from build123d import *

# Parameters (mm, degrees)
F0_W     = 60.3929003701
F0_H     = 33.9642912149
F1_DEPTH = 35.814
F2_T     = 2.54


with BuildPart() as f1:
    # F0 (on Front) → F1 (new body)
    with BuildSketch(Plane.XZ):
        with Locations((-40.0745426305, 29.1485004127)):
            Rectangle(F0_W, F0_H)
    extrude(amount=F1_DEPTH)

    # F2 (hollow, outwards: the wall grows on the outside; the body as it was is the cavity)
    f2_inside = f1.part
    offset(amount=F2_T, kind=Kind.INTERSECTION)
    add(f2_inside, mode=Mode.SUBTRACT)


solid = f1.part
Verification items for the finished model (mm, model axes). A direction names the side the tool comes from. Coordinates: 2 decimals unless noted, no trailing zeros. Order: outer loops, then holes, each group sorted by start corner. A loop starts at its lowest first (then second) coordinate and runs counter-clockwise, first axis right, second up.
Item 1: Section check B-B, the plane y = -7.5. Enter the section's corners in (x, z).
Filled in:
outline: (-72.81, 9.63) - (-7.34, 9.63) - (-7.34, 48.67) - (-72.81, 48.67) - close; hole (-70.27, 12.17) - (-9.88, 12.17) - (-9.88, 46.13) - (-70.27, 46.13) - close
Item 2: Section check A-A, the plane x = -26.5. Enter the section's corners in (y, z), then the cut area to 3 significant figures.
Filled in:
outline: (-38.35, 9.63) - (2.54, 9.63) - (2.54, 48.67) - (-38.35, 48.67) - close; hole (-35.81, 12.17) - (0, 12.17) - (0, 46.13) - (-35.81, 46.13) - close
area: 380 mm2
Item 3: Release check for a two-part mould opening along X. For faces 1 (the face through (-41, -18, 9.626)), 2 (the face through (-9.878, -18, 29)), 3 (the face through (-72.811, -18, 29)) record: +X half, -X half, draft (parallel to the pull), parting line (faces both ways), or undercut.
Filled in:
face 1: draft
face 2: undercut
face 3: -X half
Item 4: Access from +Z, -Z, +X, -X, +Y, -Y to the whole of each face (thin tool, end or side, straight path). Record for faces 4 (the face through (-41, 2.54, 29)), 5 (the face through (-70.271, -18, 29)).
Filled in:
face 4: +Z, -Z, +X, -X, +Y
face 5: none
Item 5: Material ranges on L1, parallel to Y at x = -46.5, z = 43; L2, parallel to Z at x = -59, y = -28; L3, parallel to X at y = -28, z = 28, recorded low to high.
Filled in:
L1: y = -38.35 to -35.81, 0 to 2.54
L2: z = 9.63 to 12.17, 46.13 to 48.67
L3: x = -72.81 to -70.27, -9.88 to -7.34
